Autodesk Inventor part; units mm, degrees
ref_plane "YZ Plane" through (0, 0, 0) normal (1, 0, 0) x (0, 1, 0)
ref_plane "XZ Plane" through (0, 0, 0) normal (0, 1, 0) x (-1, 0, 0)
ref_plane "XY Plane" through (0, 0, 0) normal (0, 0, 1) x (1, 0, 0)
sketch "Sketch5" plane through (0, 0, 0) normal (0, 1, 0) x (-1, 0, 0)
  circle A0 centre (0, 0) radius 15
  circle A1 centre (0, 0) radius 18
  dimension "d18" = 30
  dimension "d19" = 36
extrude "Extrusion4" add sketch "Sketch5" along normal blind 5
sketch "Sketch6" plane through (0, 0, 0) normal (0, -1, 0) x (1, 0, 0)
  circle A0 centre (0, 0) radius 15
  circle A1 centre (0, 0) radius 18
extrude "Extrusion5" add sketch "Sketch6" along normal blind 3 contours A0 | A1
sketch "Sketch7" plane through (0, 5, 0) normal (0, 1, 0) x (1, 0, 0)
  circle A0 centre (0, 0) radius 15
  circle A1 centre (0, 0) radius 18
  line L0 (-17.8255, 2.5) -> (17.8255, 2.5)
  line L1 (-17.8255, -2.5) -> (17.8255, -2.5)
  circle A2 centre (0, 0) radius 10
  line L2 (-10, 2.5) -> (-10, -2.5)
  line L3 (10, 2.5) -> (10, -2.5)
  point P0 (0, 2.5)
  point P1 (-14.7902, 2.5)
  point P2 (14.7902, 2.5)
  point P3 (14.7902, -2.5)
  point P4 (-14.7902, -2.5)
  dimension "d24" = 2.5
  dimension "d25" = 20
extrude "Extrusion6" add sketch "Sketch7" along normal blind 5 contours A0 L1 L3 L0 | A0 L0 A1 L1 | A0 L0 A1 | L1 A1 A0 | L0 L2 L1 A0 | A0 L1 A1 L0
fillet "Fillet1" radius 1.5 10 edges at (-10, 7.5, 2.5) (-10, 10, 0) (10, 7.5, 2.5) (10, 10, 0) (10, 7.5, -2.5) (-10, 7.5, -2.5) (12.3951, 10, 2.5) (12.3951, 10, -2.5) (-12.3951, 10, 2.5) (-12.3951, 10, -2.5)
sketch "Sketch8" plane through (0, 0, 0) normal (0, 1, 0) x (1, 0, 0)
  arc A0 (-10, 1) -> (-11.5, 2.5) centre (-11.5, 1) ccw
  line L0 (-11.5, 2.5) -> (-14.7902, 2.5)
  line L1 (-10, -1) -> (-10, 1)
  arc A1 (-11.5, -2.5) -> (-10, -1) centre (-11.5, -1) ccw
  line L2 (-14.7902, -2.5) -> (-11.5, -2.5)
  line L3 (11.5, -2.5) -> (14.7902, -2.5)
  arc A2 (10, -1) -> (11.5, -2.5) centre (11.5, -1) ccw
  line L4 (10, 1) -> (10, -1)
  arc A3 (11.5, 2.5) -> (10, 1) centre (11.5, 1) ccw
  line L5 (14.7902, 2.5) -> (11.5, 2.5)
  arc A4 (14.9666, 1) -> (-14.9666, 1) centre (0, 0) ccw
  line L6 (-14.7902, -3.5) -> (-11.5, -3.5)
  arc A5 (-11.5, -3.5) -> (-9, -1) centre (-11.5, -1) ccw
  line L7 (-9, -1) -> (-9, 1)
  arc A6 (-9, 1) -> (-11.5, 3.5) centre (-11.5, 1) ccw
  line L8 (-11.5, 3.5) -> (-14.7902, 3.5)
  line L9 (14.7902, -3.5) -> (11.5, -3.5)
  arc A7 (9, -1) -> (11.5, -3.5) centre (11.5, -1) ccw
  line L10 (9, -1) -> (9, 1)
  arc A8 (11.5, 3.5) -> (9, 1) centre (11.5, 1) ccw
  line L11 (11.5, 3.5) -> (14.7902, 3.5)
  circle A9 centre (0, 0) radius 15
  point P0 (14.586, 3.5)
  point P1 (14.586, -3.5)
  point P2 (-14.586, -3.5)
  point P3 (-14.586, 3.5)
  dimension "d29" = 1
  dimension "d30" = 1
extrude "Extrusion7" cut sketch "Sketch8" against normal through all contours L1 A1 L2 A9 A4 L0 A0 | A0 L0 A4 L8 A6 L7 A5 L6 A9 L2 A1 L1 | A4 L5 A3 L4 A2 L3 A9 L9 A7 L10 A8 L11 | A4 A9 L3 A2 L4 A3 L5
properties part number "Tapa"
Here's how the part is built. I have some questions about the finished solid (model axes, mm). A direction names the side the tool comes from. Give positions to 0.01 mm unless a question says otherwise; leave off trailing zeros. Write each loop counter-clockwise with the first axis right and the second up, starting at its lowest first coordinate (ties: lowest second). Pieces come first, ordered by that corner, then holes. Notation, with made-up numbers: (59, -27) -> (99, -27) arc R21 cw to (99, -7) -> close; hole circle Ø1 at (68, 54.25). An arc over 180 degrees is marked (long way). Use one line per item in the form item = value. Start each with the question number.
1. Imagine slicing it at A-A on y = -1. List the corners of the cut face in (x, z) for me, plus the area to 3 significant figures.
2. Imagine slicing it at B-B on x = -13. List the corners of the cut face in (y, z) for me.
3. Thinking about a two-plate mould opening in X: for faces 1 (the face through (-13.21, 9.55, -2.07)), 2 (the face through (13, -1, -3.5)), 3 (the face through (0, -3, 0)), which applies, +X half, -X half, draft (parallel to the pull), parting line (faces both ways), or undercut?
4. Imagine slicing it at D-D on z = 10.5. List the corners of the cut face in (x, y) for me, plus the area to 3 significant figures.
5. Will these pins go through, and if not, where does the flat tip stop? pin 1 Ø3.5 at (x, y) = (-13, -1.5) entering from +Z; pin 2 Ø1.5 at (x, y) = (12.5, -1.5) entering from -Z; pin 3 Ø2 at (y, z) = (7, -0.5) entering from +X; pin 4 Ø6 at (x, y) = (6.5, 5.5) entering from -Z.
6. On a 3-axis mill with a long thin cutter (end or side, diameter ignored), from which of +Z, -Z, +X, -X, +Y, -Y can I reach the whole of each face in a straight line? I mean faces 4 (the face through (-10.45, 9.57, -0.01)), 5 (the face through (10, -1, 3)), 6 (the face through (-12, 10, 0)), 7 (the face through (-14.826, -1.479, -2.276)). Say none if no direction works.
7. Imagine slicing it at C-C on y = 3.5. List the corners of the cut face in (x, z) for me, plus the area to 3 significant figures.
8. If I drill on L1, parallel to X at y = 4.5, z = 0; L2, parallel to X at y = 5.75, z = 0, over which ranges is the centre line in solid material (lowest first)?
Entries:
q1.outline = circle Ø36 at (0, 0); hole (-14.59, -3.5) -> (-11.5, -3.5) arc R2.5 ccw to (-9, -1) -> (-9, 1) arc R2.5 ccw to (-11.5, 3.5) -> (-14.59, 3.5) arc R15 ccw to start; hole (9, -1) arc R2.5 ccw to (11.5, -3.5) -> (14.59, -3.5) arc R15 ccw to (14.59, 3.5) -> (11.5, 3.5) arc R2.5 ccw to (9, 1) -> close
q1.area = 941 mm²
q2.outline = (-3, -12.45) -> (10, -12.45) -> (10, -7.48) -> (0, -7.48) -> (0, -3.5) -> (-3, -3.5) -> close; (-3, 3.5) -> (0, 3.5) -> (0, 7.48) -> (10, 7.48) -> (10, 12.45) -> (-3, 12.45) -> close; (5, -2.5) -> (8.5, -2.5) arc R1.5 ccw to (10, -1) -> (10, 1) arc R1.5 ccw to (8.5, 2.5) -> (5, 2.5) -> close
q3.face_1 = undercut
q3.face_2 = undercut
q3.face_3 = draft
q4.outline = (-14.62, -3) -> (14.62, -3) -> (14.62, 10) -> (10.71, 10) -> (10.71, 0) -> (-10.71, 0) -> (-10.71, 10) -> (-14.62, 10) -> close
q4.area = 166 mm²
q5.pin_1 = 14.05
q5.pin_2 = -13.64
q5.pin_3 = 18
q5.pin_4 = -17.66
q6.face_4 = +Y
q6.face_5 = +Y, -Y
q6.face_6 = +Z, -Z, +X, -X, +Y
q6.face_7 = -Y
q7.outline = circle Ø36 at (0, 0); hole circle Ø30 at (0, 0)
q7.area = 311 mm²
q8.L1 = -18 to -15, 15 to 18
q8.L2 = -18 to -10, 10 to 18
